Verification items for the finished model (mm, model axes). A direction names the side the tool comes from. Give positions to 0.01 mm unless a question says otherwise; leave off trailing zeros. Order: outer loops, then holes, each group sorted by start corner. A loop starts at its lowest first (then second) coordinate and runs counter-clockwise, first axis right, second up.
(1) Gauge pin test, flat ends, axial feed: pin 1 (5 mm diameter, centred on x = 0.5, z = 2, fed in from +Y); pin 2 (2 mm diameter, centred on x = -5.5, z = 5, fed in from -Y); pin 3 (2 mm diameter, centred on y = -0.5, z = -4, fed in from +X) (3 decimals). Record the tip position at first contact, or that the pin passes through.
(2) Access from +Z, -Z, +X, -X, +Y, -Y to the whole of each face (thin tool, end or side, straight path). Record for faces 1 (the face through (-34.925, -4, -3)), 2 (the face through (-41.12, -3.69, 6.43)).
(3) Sectioned sample at A-A on x = -27.5. Record the cut outline in (y, z) (1 decimal), plus the area to 3 significant figures.
(4) Scan lines: L1, parallel to X at y = -6, z = -1.5 (3 decimals); L2, parallel to Y at x = 5, z = 2.5; L3, parallel to Y at x = -38, z = 2.5. Record each from-to range of solid material in increasing order.
```python
from build123d import *

# Parameters (mm, degrees)
SKETCH5_R           = 4.7625
BOSS_EXTRUDE3_DEPTH = 76.2
CHAMFER1_SIZE       = 1.190625
BOSS_EXTRUDE4_DEPTH = 6.35
SKETCH8_OUTSIDE_W   = 322.79
SKETCH8_OUTSIDE_H   = 325
SKETCH8_OUTSIDE_R   = 7.14375
CUT_EXTRUDE3_DEPTH  = 83.55
CUT_EXTRUDE3_TAPER  = 60


with BuildPart() as part:
    # Sketch5 → Boss-Extrude3 (new body)
    with BuildSketch(Plane(origin=(41.275, 0, 0), x_dir=(0, 0, -1), z_dir=(1, 0, 0))):
        Circle(SKETCH5_R)
    extrude(amount=-BOSS_EXTRUDE3_DEPTH)

    # Chamfer1
    chamfer1_edges = [part.edges().sort_by_distance(p)[0] for p in [
        (41.275, 0, 4.7625),
    ]]
    chamfer(chamfer1_edges, length=CHAMFER1_SIZE)

    # Sketch11 → Revolve1 (revolve)
    with BuildSketch(Plane.XY):
        Polygon((-34.925, 4.7625), (-34.925, 0), (20.6375, 0), (15.875, 4.7625), align=None)
    revolve(axis=Axis((-34.925, 0, 0), (1, 0, 0)))

    # Sketch6 → Boss-Extrude4 (add)
    with BuildSketch(Plane.ZY.offset(34.925)):
        Polygon((7.14375, 4.124445986), (0, 8.248891971), (-7.14375, 4.124445986), (-7.14375, -4.124445986), (0, -8.248891971), (7.14375, -4.124445986), align=None)
    extrude(amount=BOSS_EXTRUDE4_DEPTH)

    # Sketch8 outside → Cut-Extrude3 (cut, through all)
    with BuildSketch(Plane.ZY.offset(41.275)):
        Rectangle(SKETCH8_OUTSIDE_W, SKETCH8_OUTSIDE_H)
        Circle(SKETCH8_OUTSIDE_R, mode=Mode.SUBTRACT)
    extrude(amount=-CUT_EXTRUDE3_DEPTH, taper=CUT_EXTRUDE3_TAPER, mode=Mode.SUBTRACT)


solid = part.part
```
Ans:
1. pin 1: stops at y = 4.76
1. pin 2: stops at y = -2.58
1. pin 3: stops at x = 41.275
2. face 1: +X
2. face 2: +Z, -X, -Y
3. outline: circle Ø9.5 at (0, 0)
3. area: 71.3 mm2
4. L1: x = -41.275 to -34.925
4. L2: y = -4.05 to 4.05
4. L3: y = -6.81 to 6.81
